Design review of the part shown in the three views and the two pictorial views. Dimensions are in mm from the part's minimum x, y and z. Give positions to 0.01 mm unless a question says otherwise; leave off trailing zeros. Loops run counter-clockwise (first coordinate to the right, second up) from the corner with the lowest first, then second, coordinate; pieces in that order, holes last.
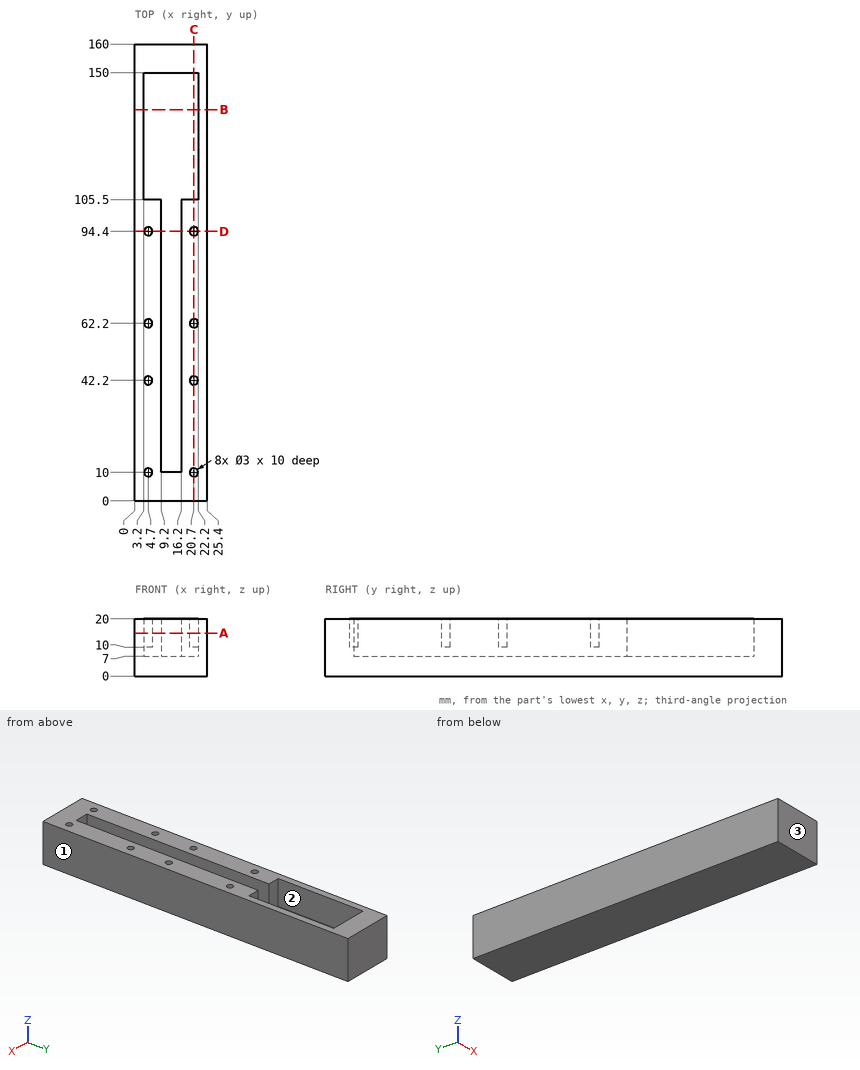
Q1. Take a section at D-D (y = 94.4). Give the boundary of the cut face in (x, z).
Results:
outline: (0, 0) - (25.4, 0) - (25.4, 20) - (22.2, 20) - (22.2, 10) - (19.2, 10) - (19.2, 20) - (16.2, 20) - (16.2, 7) - (9.2, 7) - (9.2, 20) - (6.2, 20) - (6.2, 10) - (3.2, 10) - (3.2, 20) - (0, 20) - close
Q2. Insertion check: pin 1 (1.5 mm diameter, centred on x = 21, y = 9.5, fed in from +Z); pin 2 (1 mm diameter, centred on x = 8.5, y = 140, fed in from +Z). Each pin has a flat end and moves straight along its axis. Give the tip position at first contact, or say it passes through.
Results:
pin 1: stops at z = 10
pin 2: stops at z = 7
Q3. Take a section at C-C (x = 20.7). Give the boundary of the cut face in (y, z), plus the area to 3 significant figures.
Results:
outline: (0, 0) - (160, 0) - (160, 20) - (150, 20) - (150, 7) - (105.5, 7) - (105.5, 20) - (95.9, 20) - (95.9, 10) - (92.9, 10) - (92.9, 20) - (63.7, 20) - (63.7, 10) - (60.7, 10) - (60.7, 20) - (43.7, 20) - (43.7, 10) - (40.7, 10) - (40.7, 20) - (11.5, 20) - (11.5, 10) - (8.5, 10) - (8.5, 20) - (0, 20) - close
area: 2,500 mm2
Q4. Wall thickness on line 1 (Y direction, x = 4.7, z = 14); line 2 (X direction, y = 94.4, z = 15.25); line 3 (X direction, y = 110.5, z = 10.75): over which ranges is each line inside the solid? List them lowest first.
Results:
line 1: y = 0 to 8.5, 11.5 to 40.7, 43.7 to 60.7, 63.7 to 92.9, 95.9 to 105.5, 150 to 160
line 2: x = 0 to 3.2, 6.2 to 9.2, 16.2 to 19.2, 22.2 to 25.4
line 3: x = 0 to 3.2, 22.2 to 25.4
Q5. Draft analysis for pull direction X (two halves, no side actions). For the marked faces 1, 2 and 3, state which applies: pulls with the +X half, pulls with the -X half, needs draft (parallel to the pull), parting line crosses it, or undercut.
Results:
face 1: pulls with the +X half
face 2: undercut
face 3: needs draft
Q6. Take a section at A-A (z = 15). Give the number of separate pieces and of enclosed holes in the cut face, plus the area to 3 significant figures.
Results:
separate pieces: 1
enclosed holes: 9
area: 2,490 mm2
Q7. Take a section at B-B (y = 137). Give the boundary of the cut face in (x, z), plus the area to 3 significant figures.
Results:
outline: (0, 0) - (25.4, 0) - (25.4, 20) - (22.2, 20) - (22.2, 7) - (3.2, 7) - (3.2, 20) - (0, 20) - close
area: 261 mm2
